from build123d import *

# Parameters (mm, degrees)
F2_R      = 4.653054
F3_DEPTH  = 25.4
F3_FACE_R = 4.653054
F4_DEPTH  = 97.518329


with BuildPart() as f1:
    # F0 (on Front) → F1 (revolve)
    with BuildSketch(Plane.XZ):
        with BuildLine():
            Line((-13.618723, 0), (0, 0))
            Line((0, 0), (0, 26.15414))
            Line((0, 26.15414), (-13.618723, 26.15414))
            ThreePointArc((-13.618723, 26.15414), (-37.451489, 18.678233), (-61.284255, 26.15414))
            Line((-61.284255, 26.15414), (-72.117329, 26.15414))
            Line((-72.117329, 26.15414), (-72.117329, 0))
            Line((-72.117329, 0), (-61.284255, 0))
            ThreePointArc((-61.284255, 0), (-37.451489, 8.543639), (-13.618723, 0))
        make_face()
    revolve(axis=Axis((-6.809361, 0, 26.15414), (-1, 0, 0)))

    # F2 (on face) → F3 (join)
    with BuildSketch(Plane(origin=(-72.117329, 0, 0), x_dir=(0, -1, 0), z_dir=(-1, 0, 0))):
        with Locations((0, 26.15414)):
            Circle(F2_R)
    extrude(amount=F3_DEPTH)

    # F3_face (on face) → F4 (cut, through all)
    with BuildSketch(Plane(origin=(-97.517329, 0, 26.15414), x_dir=(0, -1, 0), z_dir=(-1, 0, 0))):
        Circle(F3_FACE_R)
    extrude(amount=-F4_DEPTH, mode=Mode.SUBTRACT)


solid = f1.part
The model under review builds one solid part; all positions refer to its coordinate system, in mm. Give positions to 0.01 mm unless a question says otherwise; leave off trailing zeros. Order: outer loops, then holes, each group sorted by start corner. A loop starts at its lowest first (then second) coordinate and runs counter-clockwise, first axis right, second up. Notation, with made-up numbers: M 88.25,83 L 120.25,83 A25 ccw 120.25,96 Z; hole C -31,-35.5 d9. An arc over 180 degrees is marked long. Answer in a Markdown table with one row per item. Add a question column.
1. Add section B-B on x = -58. State the section outline as (y, z) points, plus the area to 3 significant figures.
2. To check wall thickness, follow line 1 along Z through (x, y) = (-66, 0); line 2 along Z through (x, y) = (-31, 0.5); line 3 along X through (y, z) = (11, 44). State the ranges of each line that lie inside material, in increasing order.
3. Mouldability with a two-part tool opening along Y and no side actions: class faces 1 (the cylindrical face through (-11.34, 1.01, 21.61)), 2 (the cylindrical face through (-6.714, 15.914, 46.909)), 3 (the flat face through (0, 0, 21)) as released by +Y, released by -Y, zero draft, split by the parting line, or undercut.
4. Add section A-A on x = -5. State the section outline as (y, z) points.
5. For pin 1 Ø6 at (x, y) = (-51, 7.5) entering from +Z; pin 2 Ø1 at (x, z) = (-40, 19) entering from +Y; pin 3 Ø8 at (x, z) = (-60, 37) entering from -Y, all flat-tipped, find the tip position at first contact; note any pin that passes through.
The answers:
| question | item | result |
|---|---|---|
| 1 | outline | C 0,26.15 d47.48; hole C 0,26.15 d9.31 |
| 1 | area | 1,700 mm2 |
| 2 | line 1 | 0 to 21.5, 30.81 to 52.31 |
| 2 | line 2 | 7.99 to 19.2, 33.11 to 44.32 |
| 2 | line 3 | -72.12 to -52.95, -21.95 to 0 |
| 3 | face 1 | undercut |
| 3 | face 2 | split by the parting line |
| 3 | face 3 | zero draft |
| 4 | outline | C 0,26.15 d52.31; hole C 0,26.15 d9.31 |
| 5 | pin 1 | z = 46.55 |
| 5 | pin 2 | y = 16.4 |
| 5 | pin 3 | y = -25.18 |
